Autodesk Inventor part; units mm, degrees
ref_plane "Start Plane" through (0, 0, 0) normal (0, 0, 1) x (1, 0, 0)
ref_plane "End Plane" through (0, 0, 325) normal (0, 0, 1) x (1, 0, 0)
ref_plane "YZ Plane" through (0, 0, 0) normal (1, 0, 0) x (0, 1, 0)
ref_plane "Start Plane" through (0, 0, 0) normal (0, 0, 1) x (1, 0, 0)
ref_plane "End Plane" through (0, 0, 325) normal (0, 0, 1) x (1, 0, 0)
sketch "Sketch" plane through (0, 0, 0) normal (0, 0, 1) x (1, 0, 0)
  line L0 (-10, -7) -> (-10, 7)
  line L1 (-7, 10) -> (7, 10)
  line L2 (10, 7) -> (10, -7)
  line L3 (7, -10) -> (-7, -10)
  arc A0 (-10, -7) -> (-7, -10) centre (-7, -7) ccw
  arc A1 (-7, 10) -> (-10, 7) centre (-7, 7) ccw
  arc A2 (10, 7) -> (7, 10) centre (7, 7) ccw
  arc A3 (7, -10) -> (10, -7) centre (7, -7) ccw
  line L4 (-6, 8) -> (6, 8)
  line L5 (8, 6) -> (8, -6)
  line L6 (6, -8) -> (-6, -8)
  line L7 (-8, -6) -> (-8, 6)
  line L8 (0, 14.8698) -> (0, -14.8698) construction
  line L9 (-14.8698, 0) -> (14.8698, 0) construction
  arc A4 (-8, -6) -> (-6, -8) centre (-6, -6) ccw
  arc A5 (-6, 8) -> (-8, 6) centre (-6, 6) ccw
  arc A6 (8, 6) -> (6, 8) centre (6, 6) ccw
  arc A7 (6, -8) -> (8, -6) centre (6, -6) ccw
  dimension "d7" = 3
  dimension "d10" = 20
  dimension "d11" = 20
  dimension "d12" = 2
  dimension "d15" = 10
  dimension "d16" = 10
  dimension "d19" = 2
  dimension "d20" = 2
extrude "Body" add sketch "Sketch" along normal up to surface (325 mm away) from surface at 0
sketch "Sketch3" plane through (0, 0, 0) normal (0, 0, 1) x (1, 0, 0)
  line L0 (0, 0) -> (10, 0)
ref_plane "Work Plane3" through (0, 0, 0) normal (0, -1, 0) x (1, 0, 0)
sketch "Sketch4" plane through (0, 0, 0) normal (0, -1, 0) x (1, 0, 0)
  line L0 (-2, 0) -> (12, 0)
  line L1 (-2, 325) -> (12, 325)
  dimension "d18" = 325
equation "\"d7\" = G_IR"
equation "\"d10\" = G_H"
equation "\"d11\" = G_W"
equation "\"d12\" = G_T"
equation "\"d15\" = 0.5 * d10"
equation "\"d16\" = 0.5 * d11"
equation "\"d19\" = G_T"
equation "\"d20\" = G_T"
equation "\"d3\" = G_L"
equation "\"G_W\" = 20"
equation "\"G_H\" = 20"
equation "\"G_T\" = 2"
equation "\"G_IR\" = 3"
equation "\"G_L\" = d18"
equation "\"G_OFFSET_START\" = 0"
equation "\"G_OFFSET_END\" = 0"
equation "\"d14\" = G_OFFSET_END + B_L"
equation "\"B_L\" = 325"
properties part number "DIN EN 10210-2 - 20 x 20 x 2 - 325" material "Steel, Mild"
Here's how the part is built. I have some questions about the finished solid (model axes, mm). A direction names the side the tool comes from. Round coordinates to 2 decimals unless told otherwise and drop trailing zeros. Loops run counter-clockwise (first coordinate to the right, second up) from the corner with the lowest first, then second, coordinate; pieces in that order, holes last.
1. For faces 1 (the face through (-9, 0, 0)), 2 (the face through (8, 0, 160)), which set-ups out of +Z, -Z, +X, -X, +Y, -Y let a thin tool reach every point of the face, with its end or its side?
Answers:
face 1: -Z, +X, -X, +Y, -Y
face 2: +Z, -Z
2. Thinking about a two-plate mould opening in Y: for faces 3 (the face through (0, 8, 160)), 4 (the face through (-9, 0, 325)), 5 (the face through (0, -10, 160)), which applies, released by +Y, released by -Y, zero draft, split by the parting line, or undercut?
Answers:
face 3: undercut
face 4: zero draft
face 5: released by -Y
3. Suppose I cut it at A-A, the plane y = -2. Please give me the cut outline in (x, z), and give its area (3 significant figures).
Answers:
outline: (-10, 0) - (-8, 0) - (-8, 325) - (-10, 325) - close; (8, 0) - (10, 0) - (10, 325) - (8, 325) - close
area: 1,300 mm2
4. If I drill on probe 1 along Y at (x, z) = (0.5, 54.5); probe 2 along Y at (x, z) = (-7.25, 192.5), over which ranges is the centre line in solid material (lowest first)?
Answers:
probe 1: y = -10 to -8, 8 to 10
probe 2: y = -9.99 to -7.56, 7.56 to 9.99
5. Suppose I cut it at C-C, the plane z = 143.5. Please give me the cut outline in (x, y), and give its area (3 significant figures).
Answers:
outline: (-10, -7) arc R3 ccw to (-7, -10) - (7, -10) arc R3 ccw to (10, -7) - (10, 7) arc R3 ccw to (7, 10) - (-7, 10) arc R3 ccw to (-10, 7) - close; hole (-8, -6) arc R2 ccw to (-6, -8) - (6, -8) arc R2 ccw to (8, -6) - (8, 6) arc R2 ccw to (6, 8) - (-6, 8) arc R2 ccw to (-8, 6) - close
area: 140 mm2
